Can you work these out from the model? Positions are in its coordinate system, mm. A direction names the side the tool comes from. Round coordinates to 2 decimals unless told otherwise and drop trailing zeros. Loops run counter-clockwise (first coordinate to the right, second up) from the corner with the lowest first, then second, coordinate; pieces in that order, holes last. Notation, with made-up numbers: (-38.5, 54) - (-17.5, 54) arc R19 ccw to (-17.5, 77) - close; hole circle Ø5 at (6, 52.25). An arc over 180 degrees is marked (long way). Answer as CSV lines item,"result".
```python
from build123d import *

# Parameters (mm, degrees)
SKETCH021_R          = 33
PAD018_DEPTH         = 12.5
PAD018_DEPTH_BACK    = 12.5
SKETCH_004_R         = 6
POCKET021_DEPTH      = 20
POCKET021_DEPTH_BACK = 20
SKETCH035_W          = 175.5
SKETCH035_H          = 210
POCKET022_DEPTH      = 20
POCKET022_DEPTH_BACK = 20


with BuildPart() as part:
    # Sketch021 → Pad018 (new body, two sides)
    with BuildSketch(Plane.XY) as pad018_sk:
        with BuildLine():
            Line((-110, -105), (110, -105))
            Line((110, -105), (120.90162, -105))
            ThreePointArc((120.90162, -105), (127.335146, -102.335146), (130, -95.90162))
            Line((130, -95.90162), (130, -89.09838))
            ThreePointArc((130, -89.09838), (127.335146, -82.664854), (120.90162, -80))
            Line((120.90162, -80), (119.09838, -80))
            ThreePointArc((110, -70.90162), (112.664854, -77.335146), (119.09838, -80))
            Line((110, -70.90162), (110, 0))
            Line((110, 70.90162), (110, 0))
            ThreePointArc((119.09838, 80), (112.664854, 77.335146), (110, 70.90162))
            Line((120.90162, 80), (119.09838, 80))
            ThreePointArc((120.90162, 80), (127.335146, 82.664854), (130, 89.09838))
            Line((130, 95.90162), (130, 89.09838))
            ThreePointArc((130, 95.90162), (127.335146, 102.335146), (120.90162, 105))
            Line((110, 105), (120.90162, 105))
            Line((110, 105), (-110, 105))
            Line((-110, 105), (-110, 0))
            Line((-110, -105), (-110, 0))
        make_face()
        Circle(SKETCH021_R, mode=Mode.SUBTRACT)
    extrude(amount=-PAD018_DEPTH)
    extrude(pad018_sk.sketch, amount=PAD018_DEPTH_BACK)

    # Sketch_004 → Pocket021 (cut, two sides)
    with BuildSketch(Plane.XY) as pocket021_sk:
        with Locations((-118, 93)):
            Circle(SKETCH_004_R)
        with Locations((118, 93)):
            Circle(SKETCH_004_R)
        with Locations((-118, -93)):
            Circle(SKETCH_004_R)
        with Locations((118, -93)):
            Circle(SKETCH_004_R)
        with BuildLine():
            ThreePointArc((86.75, 75), (87.81066, 75.43934), (88.25, 76.5))
            Line((88.25, 105), (88.25, 76.5))
            Line((88.25, 105), (6.75, 105))
            Line((6.75, 105), (6.75, 76.5))
            ThreePointArc((6.75, 76.5), (7.18934, 75.43934), (8.25, 75))
            Line((86.75, 75), (8.25, 75))
        make_face()
        with BuildLine():
            ThreePointArc((-88.25, 76.5), (-87.81066, 75.43934), (-86.75, 75))
            Line((-86.75, 75), (-8.25, 75))
            ThreePointArc((-8.25, 75), (-7.18934, 75.43934), (-6.75, 76.5))
            Line((-6.75, 105), (-6.75, 76.5))
            Line((-88.25, 105), (-6.75, 105))
            Line((-88.25, 105), (-88.25, 76.5))
        make_face()
        with BuildLine():
            ThreePointArc((88.25, -76.5), (87.81066, -75.43934), (86.75, -75))
            Line((86.75, -75), (8.25, -75))
            ThreePointArc((8.25, -75), (7.18934, -75.43934), (6.75, -76.5))
            Line((6.75, -105), (6.75, -76.5))
            Line((88.25, -105), (6.75, -105))
            Line((88.25, -105), (88.25, -76.5))
        make_face()
        with BuildLine():
            ThreePointArc((-86.75, -75), (-87.81066, -75.43934), (-88.25, -76.5))
            Line((-88.25, -105), (-88.25, -76.5))
            Line((-88.25, -105), (-6.75, -105))
            Line((-6.75, -105), (-6.75, -76.5))
            ThreePointArc((-6.75, -76.5), (-7.18934, -75.43934), (-8.25, -75))
            Line((-86.75, -75), (-8.25, -75))
        make_face()
    extrude(amount=-POCKET021_DEPTH, mode=Mode.SUBTRACT)
    extrude(pocket021_sk.sketch, amount=POCKET021_DEPTH_BACK, mode=Mode.SUBTRACT)

    # Sketch035 → Pocket022 (cut, two sides)
    with BuildSketch(Plane.XY) as pocket022_sk:
        with Locations((-22.25, 0)):
            Rectangle(SKETCH035_W, SKETCH035_H)
    extrude(amount=-POCKET022_DEPTH, mode=Mode.SUBTRACT)
    extrude(pocket022_sk.sketch, amount=POCKET022_DEPTH_BACK, mode=Mode.SUBTRACT)


solid = part.part
```
Q1. Imagine slicing it at D-D (y = 16). Write out the boundary of the cut face in (x, z).
Checks:
outline,"(65.5, -12.5) - (110, -12.5) - (110, 12.5) - (65.5, 12.5) - close"
Q2. We'd pull the mould along X, two halves only. Please class faces 1 (the cylindrical face through (127.41, 102.26, -0.18)), 2 (the flat face through (90, 1, -12.5)), 3 (the cylindrical face through (113.58, -88.94, 0.18)): pulls with the +X half, pulls with the -X half, needs draft (parallel to the pull), parting line crosses it, or undercut.
Checks:
face 1,"pulls with the +X half"
face 2,"needs draft"
face 3,"undercut"
Q3. On a 3-axis mill with a long thin cutter (end or side, diameter ignored), from which of +Z, -Z, +X, -X, +Y, -Y can I reach the whole of each face in a straight line? I mean faces 4 (the flat face through (65.5, -1, 0)), 5 (the flat face through (76, -75, 0)), 6 (the flat face through (76, 75, 0)), 7 (the cylindrical face through (112.74, 77.41, -0.18)). Say none if no direction works.
Checks:
face 4,"+Z, -Z, -X, +Y, -Y"
face 5,"+Z, -Z, -X, -Y"
face 6,"+Z, -Z, -X, +Y"
face 7,"+Z, -Z, +X"
Q4. Imagine slicing it at A-A (y = 93). Write out the boundary of the cut face in (x, z), then the cut area to 3 significant figures.
Checks:
outline,"(88.25, -12.5) - (112, -12.5) - (112, 12.5) - (88.25, 12.5) - close; (124, -12.5) - (130, -12.5) - (130, 12.5) - (124, 12.5) - close"
area,"744 mm²"
Q5. Imagine slicing it at C-C (x = 116.5). Write out the boundary of the cut face in (y, z), then the cut area to 3 significant figures.
Checks:
outline,"(-105, -12.5) - (-98.81, -12.5) - (-98.81, 12.5) - (-105, 12.5) - close; (-87.19, -12.5) - (-79.62, -12.5) - (-79.62, 12.5) - (-87.19, 12.5) - close; (79.62, -12.5) - (87.19, -12.5) - (87.19, 12.5) - (79.62, 12.5) - close; (98.81, -12.5) - (105, -12.5) - (105, 12.5) - (98.81, 12.5) - close"
area,"688 mm²"
Q6. If I drill on line 1 along X through (y, z) = (-93, -6); line 2 along Y through (x, z) = (118, -6.25); line 3 along Y through (x, z) = (123, -6.25), over which ranges is the centre line in solid material (lowest first)? Write a range as [from, to].
Checks:
line 1,"[88.25, 112], [124, 130]"
line 2,"[-105, -99], [-87, -79.93], [79.93, 87], [99, 105]"
line 3,"[-104.75, -96.32], [-89.68, -80.25], [80.25, 89.68], [96.32, 104.75]"
Q7. Imagine slicing it at B-B (z = 2.5). Write out the boundary of the cut face in (x, y).
Checks:
outline,"(65.5, -75) - (86.75, -75) arc R1.5 cw to (88.25, -76.5) - (88.25, -105) - (120.9, -105) arc R9.1 ccw to (130, -95.9) - (130, -89.1) arc R9.1 ccw to (120.9, -80) - (119.1, -80) arc R9.1 cw to (110, -70.9) - (110, 70.9) arc R9.1 cw to (119.1, 80) - (120.9, 80) arc R9.1 ccw to (130, 89.1) - (130, 95.9) arc R9.1 ccw to (120.9, 105) - (88.25, 105) - (88.25, 76.5) arc R1.5 cw to (86.75, 75) - (65.5, 75) - close; hole circle Ø12 at (118, -93); hole circle Ø12 at (118, 93)"
Q8. I'm going to push flat-ended pins straight in: pin 1 Ø1.5 at (x, z) = (84.5, 8.5) entering from -Y; pin 2 Ø10.5 at (x, z) = (74, -0.5) entering from +Y; pin 3 Ø8 at (y, z) = (47.5, 5.5) entering from +X; pin 4 Ø19 at (x, y) = (118, 93) entering from +Z. Where does each tip first touch, or does it pass through?
Checks:
pin 1,"y = -75"
pin 2,"y = 75"
pin 3,"x = 110"
pin 4,"z = 12.5"
